```python
from build123d import *

# Parameters (mm, degrees)
ESBO_O1_R                = 1.75
RESSALTO_EXTRUS_O1_DEPTH = 3


with BuildPart() as part:
    # Esboço1 → Ressalto-extrusão1 (new body)
    # profile 1 of 3: a face of its own
    with BuildSketch(Plane.XY):
        with BuildLine():
            ThreePointArc((0, 5), (-5, 0), (0, -5))
            Line((0, -5), (-20, -5))
            Line((-20, -5), (-20, 5))
            Line((-20, 5), (0, 5))
        make_face()
        with Locations((-17, -2)):
            Circle(ESBO_O1_R, mode=Mode.SUBTRACT)
        with Locations((-13, 2)):
            Circle(ESBO_O1_R, mode=Mode.SUBTRACT)
    # profile 2 of 3: a face of its own
    with BuildSketch(Plane.XY):
        with BuildLine():
            ThreePointArc((75.044247788, -70.663716814), (49.858206024, -23.733478829), (0, -5))
            Line((0, -5), (0, 5))
            ThreePointArc((0, 5), (56.443252103, -16.207711882), (84.955752212, -69.336283186))
            ThreePointArc((84.955752212, -69.336283186), (80.663716814, -74.955752212), (75.044247788, -70.663716814))
        make_face()
        with Locations((80, -70)):
            Circle(ESBO_O1_R, mode=Mode.SUBTRACT)
    # profile 3 of 3: a face of its own
    with BuildSketch(Plane.XY):
        with BuildLine():
            Line((0, 5), (0, -5))
            ThreePointArc((0, -5), (-5, 0), (0, 5))
        make_face()
    extrude(amount=RESSALTO_EXTRUS_O1_DEPTH)


solid = part.part
```
Here's how the part is built. I have some questions about the finished solid (model axes, mm). A direction names the side the tool comes from. Round coordinates to 2 decimals unless told otherwise and drop trailing zeros. Order: outer loops, then holes, each group sorted by start corner. A loop starts at its lowest first (then second) coordinate and runs counter-clockwise, first axis right, second up. Notation, with made-up numbers: M 36,-27.5 L 64,-27.5 A18 ccw 64,-5.5 Z; hole C -13.75,32 d3. An arc over 180 degrees is marked long. Answer as CSV lines item,"result".
Item 1: We'd pull the mould along Y, two halves only. Please class faces 1 (the cylindrical face through (50.43, -24.24, 1.48)), 2 (the flat face through (-20, 0, 1)), 3 (the cylindrical face through (81.617, -70.67, 1.479)): +Y half, -Y half, draft (parallel to the pull), parting line (faces both ways), or undercut.
From the geometry:
face 1,"-Y half"
face 2,"draft"
face 3,"undercut"
Item 2: Imagine slicing it at A-A on x = -13. List the corners of the cut face in (y, z) for me.
From the geometry:
outline,"M -5,0 L 0.25,0 L 0.25,3 L -5,3 Z; M 3.75,0 L 5,0 L 5,3 L 3.75,3 Z"
Item 3: Imagine slicing it at C-C on y = -2. List the corners of the cut face in (x, z) for me, and give its area (3 significant figures).
From the geometry:
outline,"M -20,0 L -18.75,0 L -18.75,3 L -20,3 Z; M -15.25,0 L 33.93,0 L 33.93,3 L -15.25,3 Z"
area,"151 mm2"
Item 4: Which directions (+Z, -Z, +X, -X, +Y, -Y) give clear straight access to the entire face, cutting with the end or side of a thin tool? Please do faces 4 (the flat face through (-10, -5, 1)), 5 (the flat face through (-10, 5, 1)).
From the geometry:
face 4,"+Z, -Z, -X, -Y"
face 5,"+Z, -Z, +X, -X, +Y"
Item 5: For pin 1 (4 mm diameter, centred on x = 80, y = -70, fed in from -Z); pin 2 (1 mm diameter, centred on x = 41.5, z = 0.5, fed in from -Y); pin 3 (1 mm diameter, centred on y = -40, z = 0.5, fed in from +X); pin 4 (1.5 mm diameter, centred on y = -26.5, z = 0.5, fed in from -X), each with a flat end and sliding along its axis, tell me the tip position at first contact or that it passes through.
From the geometry:
pin 1,"z = 0"
pin 2,"y = -17.72"
pin 3,"x = 75.7"
pin 4,"x = 52.07"
Item 6: Please list where these lines run through material, in increasing order: L1, parallel to Y at x = -17, z = 2.2; L2, parallel to Y at x = -13, z = 1.25; L3, parallel to Y at x = 20.5, z = 1.5. Write a range as [from, to].
From the geometry:
L1,"[-5, -3.75], [-0.25, 5]"
L2,"[-5, 0.25], [3.75, 5]"
L3,"[-7.83, 2.51]"
Item 7: Imagine slicing it at D-D on x = 46. List the corners of the cut face in (y, z) for me, and give its area (3 significant figures).
From the geometry:
outline,"M -20.58,0 L -8.39,0 L -8.39,3 L -20.58,3 Z"
area,"36.6 mm2"
Item 8: Imagine slicing it at B-B on z = 0.5. List the corners of the cut face in (x, y) for me, and give its area (3 significant figures).
From the geometry:
outline,"M -20,-5 L 0,-5 A75.71 cw 75.04,-70.66 A5 ccw 84.96,-69.34 A85.71 ccw 0,5 L -20,5 Z; hole C -17,-2 d3.5; hole C -13,2 d3.5; hole C 80,-70 d3.5"
area,"1,370 mm2"
